Here's how the part is built. I have some questions about the finished solid (model axes, mm). Face numbers are marked on the shaded views. Round coordinates to 2 decimals unless told otherwise and drop trailing zeros. Order: outer loops, then holes, each group sorted by start corner. A loop starts at its lowest first (then second) coordinate and runs counter-clockwise, first axis right, second up.
```python
from build123d import *

# Parameters (mm, degrees)
F0_R      = 19.1485137608
F1_DEPTH  = 76.2
F2_R      = 10.1427054409
F3_DEPTH  = 76.2
F4_W      = 38.1332449615
F4_H      = 16.2587165833
F5_DEPTH  = 76.2
F6_W      = 38.222245872
F6_H      = 13.4063065052
F7_DEPTH  = 76.2
F9_DEPTH  = 127
F11_DEPTH = 127
F12_R     = 9.6381691068
F13_DEPTH = 127


with BuildPart() as f1:
    # F0 (on Front) → F1 (new body)
    with BuildSketch(Plane.XZ):
        Circle(F0_R)
    extrude(amount=F1_DEPTH)

    # F2 (on face) → F3 (cut)
    with BuildSketch(Plane.XZ.offset(76.2)):
        Circle(F2_R)
    extrude(amount=-F3_DEPTH, mode=Mode.SUBTRACT)

    # F4 (on Top) → F5 (join)
    with BuildSketch(Plane.XY):
        with Locations((0, -8.1293582916)):
            Rectangle(F4_W, F4_H)
    extrude(amount=F5_DEPTH)

    # F6 (on Top) → F7 (join)
    with BuildSketch(Plane.XY):
        with Locations((0, -69.3134739995)):
            Rectangle(F6_W, F6_H)
    extrude(amount=F7_DEPTH)

    # F8 (on face) → F9 (cut)
    with BuildSketch(Plane.XZ.offset(76.0166272521)):
        with BuildLine():
            ThreePointArc((10.1427054409, 0), (0, 10.1427054409), (-10.1427054409, 0))
            Line((-10.1427054409, 0), (10.1427054409, 0))
        make_face()
    extrude(amount=-F9_DEPTH, mode=Mode.SUBTRACT)

    # F10 (on face) → F11 (cut)
    with BuildSketch(Plane.XZ.offset(76.0166272521)):
        with BuildLine():
            ThreePointArc((-19.111122936, 56.6924431661), (0, 75.16739223), (19.111122936, 56.6924431661))
            Line((19.111122936, 56.6924431661), (19.111122936, 76.2))
            Line((19.111122936, 76.2), (-19.111122936, 76.2))
            Line((-19.111122936, 76.2), (-19.111122936, 56.6924431661))
        make_face()
    extrude(amount=-F11_DEPTH, mode=Mode.SUBTRACT)

    # F12 (on face) → F13 (cut)
    with BuildSketch(Plane.XZ.offset(76.0166272521)):
        with Locations((0, 58.5922114551)):
            Circle(F12_R)
    extrude(amount=-F13_DEPTH, mode=Mode.SUBTRACT)


solid = f1.part
```
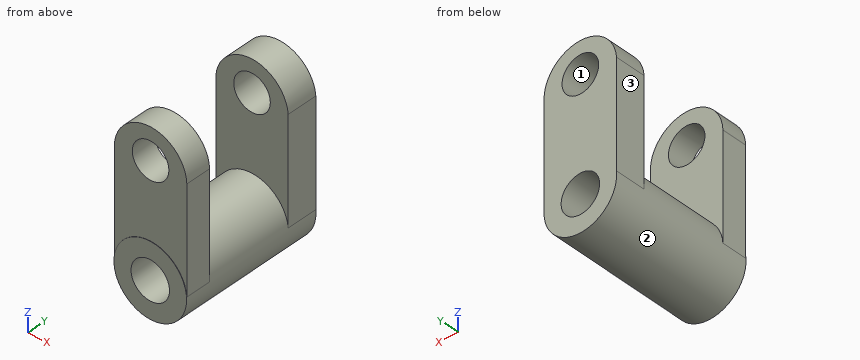
1. I'm going to push flat-ended pins straight in: P1, Ø10, axis at x = 10, y = -16, coming from the -Z side; P2, Ø22, axis at x = 0, z = 58.59, coming from the -Y side; P3, Ø8, axis at x = -5, y = -55, coming from the -Z side. Where does each tip first touch, or does it pass through?
Evaluation:
P1: stops at z = -18.48
P2: stops at y = -76.02
P3: stops at z = -19.12
2. I need wall thicknesses on probe 1 along Z at (x, y) = (0, -67.5); probe 2 along Y at (x, z) = (13, 27.5); probe 3 along Z at (x, y) = (0, -36). Which ranges of each line are inside material? Lowest first, please.
Evaluation:
probe 1: z = -19.15 to -10.14, 10.14 to 48.95, 68.23 to 75.17
probe 2: y = -76.02 to -62.61, -16.26 to 0
probe 3: z = -19.15 to -10.14, 10.14 to 19.15
3. If we mould it in two halves opening along Z, with no side actions, what happens to the marked faces 1, 2 and 3? For each: released by +Z, released by -Z, zero draft, split by the parting line, or undercut.
Evaluation:
face 1: undercut
face 2: split by the parting line
face 3: zero draft
4. If we section it at B-B, the plane x = 0: Write out the boundary of the cut face in (y, z), and give its area (3 significant figures).
Evaluation:
outline: (-76.2, -19.15) - (0, -19.15) - (0, -10.14) - (-76.2, -10.14) - close; (-76.2, 10.14) - (0, 10.14) - (0, 48.95) - (-16.26, 48.95) - (-16.26, 19.15) - (-62.61, 19.15) - (-62.61, 48.95) - (-76.02, 48.95) - (-76.02, 19.15) - (-76.2, 19.15) - close; (-76.02, 68.23) - (-62.61, 68.23) - (-62.61, 75.17) - (-76.02, 75.17) - close; (-16.26, 68.23) - (0, 68.23) - (0, 75.17) - (-16.26, 75.17) - close
area: 2,460 mm2
5. If we section it at C-C, the plane y = -23: Write out the boundary of the cut face in (x, z).
Evaluation:
outline: circle Ø38.3 at (0, 0); hole circle Ø20.29 at (0, 0)
6. If we section it at A-A, the plane z = 0: Write out the boundary of the cut face in (x, y).
Evaluation:
outline: (-19.15, -76.2) - (-10.14, -76.2) - (-10.14, 0) - (-19.15, 0) - close; (10.14, -76.2) - (19.15, -76.2) - (19.15, 0) - (10.14, 0) - close
7. If we section it at D-D, the plane z = 31: Write out the boundary of the cut face in (x, y).
Evaluation:
outline: (-19.11, -76.02) - (19.11, -76.02) - (19.11, -62.61) - (-19.11, -62.61) - close; (-19.07, -16.26) - (19.07, -16.26) - (19.07, 0) - (-19.07, 0) - close
